The listing builds one solid part. Answer for the finished solid, in the listing's coordinates (mm). Round coordinates to 2 decimals unless told otherwise and drop trailing zeros. Write each loop counter-clockwise with the first axis right and the second up, starting at its lowest first coordinate (ties: lowest second). Pieces come first, ordered by that corner, then holes. Notation, with made-up numbers: (46, 69) - (68, 69) arc R14 ccw to (68, 73) - close; hole circle Ø2 at (32.25, 75). An arc over 180 degrees is marked (long way). Answer as CSV lines item,"result". Start each with the question number.
Item 1: A cutting plane is placed at A-A on z = 3.75. Determine the outline of the cut face in (x, y), and give its area (3 significant figures).
Item 2: A cutting plane is placed at C-C on y = 2.3. Determine the outline of the cut face in (x, z) (3 decimals).
Item 3: A cutting plane is placed at B-B on x = 0. Determine the outline of the cut face in (y, z) (1 decimal).
Item 4: A cutting plane is placed at D-D on z = 0. Determine the outline of the cut face in (x, y).
Item 5: Straight lines are drawn through the part: line 1 along Y through (x, z) = (0, -3); line 2 along X through (y, z) = (-0.55, 0); line 3 along X through (y, z) = (-1.2, 0). For each, find the intervals that lie inside material, in ascending order. Write a range as [from, to].
Item 6: For a pull along Z with two mould halves and no side action, classify faces 1 (the cylindrical face through (-0.966, 0.013, -1.26)), 2 (the flat face through (-2, -0.953, 1)), 3 (the flat face through (0, -2, 4.445)), 4 (the cylindrical face through (1.26, 0.04, -0.17)) as pulls with the +Z half, pulls with the -Z half, needs draft (parallel to the pull), parting line crosses it, or undercut.
Item 7: A flat-ended cylindrical pin translates along its axis: pin 1 (1.5 mm diameter, centred on x = 0, z = 0, fed in from +Y). Find the tip coordinate at first contact, or state that the pin passes through.
```python
from build123d import *

# Parameters (mm, degrees)
SKETCH3_R           = 1.5875
BOSS_EXTRUDE2_DEPTH = 2.7305
SKETCH4_W           = 6.604
SKETCH4_H           = 8.89
BOSS_EXTRUDE3_DEPTH = 1.778
SKETCH5_W           = 6.604
SKETCH5_H           = 8.89
BOSS_EXTRUDE4_DEPTH = 1.778
SKETCH6_R           = 1.27
CUT_EXTRUDE1_DEPTH  = 8.777129933


with BuildPart() as part:
    # Sketch3 → Boss-Extrude2 (new, symmetric)
    with BuildSketch(Plane(origin=(0, 0, 0), x_dir=(1, 0, 0), z_dir=(0, 1, 0))):
        with Locations(Location((0, 0, 0), (0, 0, 270))):
            Circle(SKETCH3_R)
    extrude(amount=BOSS_EXTRUDE2_DEPTH, both=True)

    # Sketch4 → Boss-Extrude3 (add)
    with BuildSketch(Plane.XZ.offset(2.7305)):
        Rectangle(SKETCH4_W, SKETCH4_H)
    extrude(amount=-BOSS_EXTRUDE3_DEPTH)

    # Sketch5 → Boss-Extrude4 (add)
    with BuildSketch(Plane(origin=(0, 2.7305, 0), x_dir=(1, 0, 0), z_dir=(0, 1, 0))):
        Rectangle(SKETCH5_W, SKETCH5_H)
    extrude(amount=-BOSS_EXTRUDE4_DEPTH)

    # Sketch6 → Cut-Extrude1 (cut, through all)
    with BuildSketch(Plane(origin=(0, 2.7305, 0), x_dir=(1, 0, 0), z_dir=(0, 1, 0))):
        with Locations(Location((0, 0, 0), (0, 0, 270))):
            Circle(SKETCH6_R)
    extrude(amount=-CUT_EXTRUDE1_DEPTH, mode=Mode.SUBTRACT)


solid = part.part
```
Geometry says:
1,outline,"(-3.3, -2.73) - (3.3, -2.73) - (3.3, -0.95) - (-3.3, -0.95) - close; (-3.3, 0.95) - (3.3, 0.95) - (3.3, 2.73) - (-3.3, 2.73) - close"
1,area,"23.5 mm^2"
2,outline,"(-3.302, -4.445) - (3.302, -4.445) - (3.302, 4.445) - (-3.302, 4.445) - close; hole circle Ø2.54 at (0, 0)"
3,outline,"(-2.7, -4.4) - (-1, -4.4) - (-1, -1.6) - (1, -1.6) - (1, -4.4) - (2.7, -4.4) - (2.7, -1.3) - (-2.7, -1.3) - close; (-2.7, 1.3) - (2.7, 1.3) - (2.7, 4.4) - (1, 4.4) - (1, 1.6) - (-1, 1.6) - (-1, 4.4) - (-2.7, 4.4) - close"
4,outline,"(-3.3, -2.73) - (-1.27, -2.73) - (-1.27, 2.73) - (-3.3, 2.73) - (-3.3, 0.95) - (-1.59, 0.95) - (-1.59, -0.95) - (-3.3, -0.95) - close; (1.27, -2.73) - (3.3, -2.73) - (3.3, -0.95) - (1.59, -0.95) - (1.59, 0.95) - (3.3, 0.95) - (3.3, 2.73) - (1.27, 2.73) - close"
5,line 1,"y = [-2.73, -0.95], [0.95, 2.73]"
5,line 2,"x = [-1.59, -1.27], [1.27, 1.59]"
5,line 3,"x = [-3.3, -1.27], [1.27, 3.3]"
6,face 1,"parting line crosses it"
6,face 2,"needs draft"
6,face 3,"pulls with the +Z half"
6,face 4,"undercut"
7,pin 1,"passes through"
